Drawing for the job (mm, zero at the part's lowest x, y, z). A direction names the side the tool comes from. Round coordinates to 2 decimals unless told otherwise and drop trailing zeros. Write each loop counter-clockwise with the first axis right and the second up, starting at its lowest first coordinate (ties: lowest second). Pieces come first, ordered by that corner, then holes.
Item 1: Band-saw the part on B-B, the plane z = 1. Write the cut outline in (x, y).
Item 2: Band-saw the part on D-D, the plane y = 5.5. Write the cut outline in (x, z), then the cut area to 3 significant figures.
Item 3: Band-saw the part on A-A, the plane x = 2.5. Write the cut outline in (y, z), then the cut area to 3 significant figures.
Item 4: Drop flat-ended pins along their axis: pin 1 Ø3 at (x, z) = (15.5, 2) entering from +Y; pin 2 Ø3 at (x, z) = (10.5, 5) entering from -Y; pin 3 Ø6 at (y, z) = (9, 6.5) entering from -X; pin 4 Ø2 at (y, z) = (5.5, 9) entering from +X. Give the stop position or say it passes through.
Item 5: Band-saw the part on C-C, the plane x = 17. Write the cut outline in (y, z).
Item 6: Wall check: probe 1 along X at (y, z) = (17.25, 5.9); probe 2 along Y at (x, z) = (25, 2); probe 3 along X at (y, z) = (4.25, 2.5). Give the ranges that are in metal, low to high.
Item 7: 3-axis set-ups, long thin cutter, end or side, ignore diameter. For the marked faces 1, 2 and 3: which of +Z, -Z, +X, -X, +Y, -Y reach the whole face in a straight line?
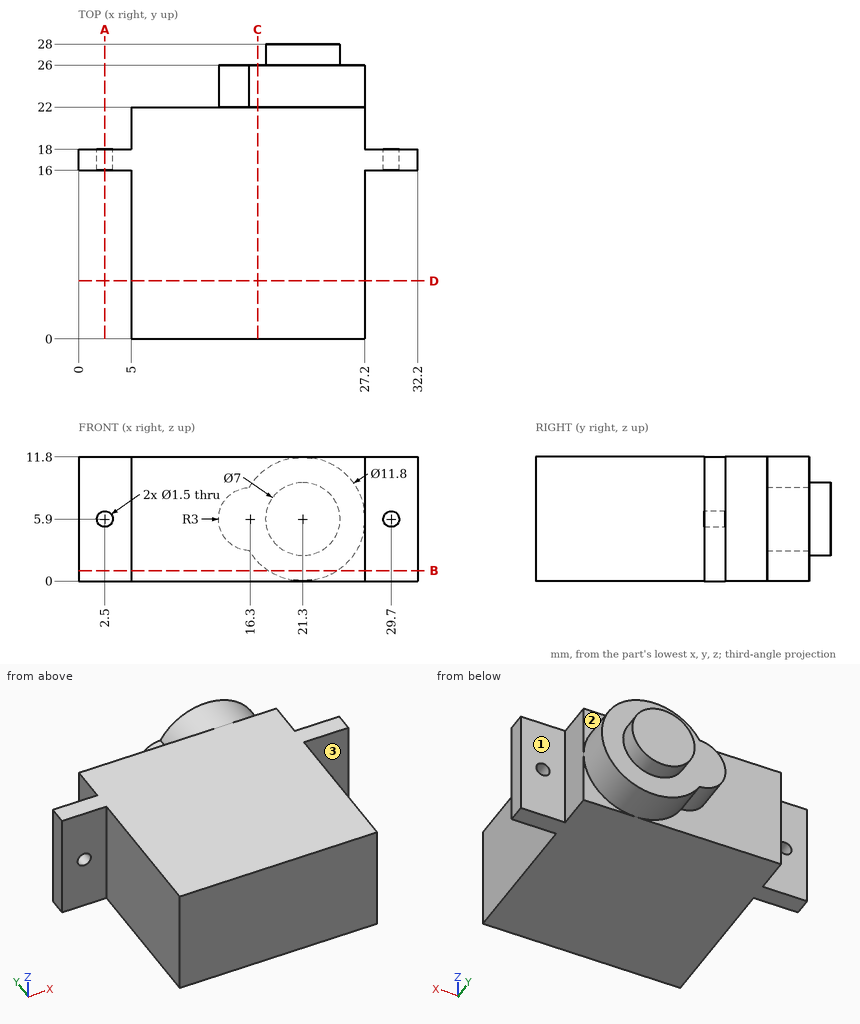
Results:
1. outline: (0, 16) - (5, 16) - (5, 0) - (27.2, 0) - (27.2, 16) - (32.2, 16) - (32.2, 18) - (27.2, 18) - (27.2, 22) - (24.59, 22) - (24.59, 26) - (18.01, 26) - (18.01, 22) - (5, 22) - (5, 18) - (0, 18) - close
2. outline: (5, 0) - (27.2, 0) - (27.2, 11.8) - (5, 11.8) - close
2. area: 262 mm2
3. outline: (16, 0) - (18, 0) - (18, 5.15) - (16, 5.15) - close; (16, 6.65) - (18, 6.65) - (18, 11.8) - (16, 11.8) - close
3. area: 20.6 mm2
4. pin 1: stops at y = 26
4. pin 2: stops at y = 0
4. pin 3: stops at x = 5
4. pin 4: stops at x = 27.2
5. outline: (0, 0) - (22, 0) - (22, 1.86) - (26, 1.86) - (26, 9.94) - (22, 9.94) - (22, 11.8) - (0, 11.8) - close
6. probe 1: x = 0 to 1.75, 3.25 to 28.95, 30.45 to 32.2
6. probe 2: y = 0 to 26
6. probe 3: x = 5 to 27.2
7. face 1: +Z, -Z, +X, +Y
7. face 2: +Z, +X, +Y
7. face 3: +Z, -Z, +X, -Y
